```python
from build123d import *

# Parameters (mm, degrees)
SKETCH_1_R          = 3
EXTRUDE_1_DEPTH     = 0.5
SKETCH_2_R          = 1.5
EXTRUDE_2_DEPTH     = 25
CHAMFER_1_SIZE      = 0.2
CUT_EXTRUDE_1_DEPTH = 0.8
FILLET_2_R          = 0.3


with BuildPart() as part:
    # 草图1 → 凸台-拉伸1 (new body, symmetric)
    with BuildSketch(Plane.XY):
        Circle(SKETCH_1_R)
    extrude(amount=EXTRUDE_1_DEPTH, both=True)

    # 草图2 → 凸台-拉伸2 (add)
    with BuildSketch(Plane(origin=(0, 0, -0.5), x_dir=(-1, 0, 0), z_dir=(0, 0, -1))):
        Circle(SKETCH_2_R)
    extrude(amount=EXTRUDE_2_DEPTH)

    # 倒角1
    chamfer_1_edges = [part.edges().sort_by_distance(p)[0] for p in [
        (1.5, 0, -25.5),
    ]]
    chamfer(chamfer_1_edges, length=CHAMFER_1_SIZE)

    # 草图3 → 切除-拉伸1 (cut)
    with BuildSketch(Plane.XY.offset(0.5)):
        Polygon((1.154700538, 0), (0.577350269, 1), (-0.577350269, 1), (-1.154700538, 0), (-0.577350269, -1), (0.577350269, -1), align=None)
    extrude(amount=-CUT_EXTRUDE_1_DEPTH, mode=Mode.SUBTRACT)

    # 圆角2
    fillet_2_edges = [part.edges().sort_by_distance(p)[0] for p in [
        (-3, 0, -0.5),
        (-3, 0, 0.5),
    ]]
    fillet(fillet_2_edges, radius=FILLET_2_R)


solid = part.part
```
The model under review builds one solid part; all positions refer to its coordinate system, in mm. A direction names the side the tool comes from. Coordinates: 2 decimals unless noted, no trailing zeros. Write each loop counter-clockwise with the first axis right and the second up, starting at its lowest first coordinate (ties: lowest second). Pieces come first, ordered by that corner, then holes.
1) We need section B-B on z = -11.5. State the section outline as (x, y) points.
2) Machinability: for faces 4 (the face through (1.2, -1.2, -0.5)), 5 (the face through (0, -1.2, 0.5)), which of the approach directions +Z, -Z, +X, -X, +Y, -Y give a long, thin tool a straight path to every point of the face, cutting with its end or side? Answer none if there is none.
3) We need section A-A on x = 0. State the section outline as (y, z) points, then the cut area to 3 significant figures.
4) Clearance check with flat-ended pins moving along their axes: pin 1 Ø0.6 at (x, y) = (-0.5, 0) entering from +Z; pin 2 Ø1 at (x, z) = (1, -10.5) entering from -Y; pin 3 Ø1 at (y, z) = (-1.5, -17) entering from +X. State where each tip first meets the part, or that it passes through.
5) To check wall thickness, follow probe 1 along Z at (x, y) = (-1.5, 2.25); probe 2 along X at (y, z) = (0.75, -2.25); probe 3 along Z at (x, y) = (1.5, 2.5). State the ranges of each line that lie inside material, in increasing order.
6) The part is to be moulded in two halves that separate along X. For faces 1 (the face through (1.5, 0.07, -12.73)), 2 (the face through (0, 0, -25.5)), 3 (the face through (0, 0, -0.3)), say which applies: pulls with the +X half, pulls with the -X half, needs draft (parallel to the pull), parting line crosses it, or undercut.
Answer list:
1. outline: circle Ø3 at (0, 0)
2. face 4: -Z
2. face 5: +Z, +X, -X, +Y, -Y
3. outline: (-3, -0.2) arc R0.3 ccw to (-2.7, -0.5) - (-1.5, -0.5) - (-1.5, -25.3) - (-1.3, -25.5) - (1.3, -25.5) - (1.5, -25.3) - (1.5, -0.5) - (2.7, -0.5) arc R0.3 ccw to (3, -0.2) - (3, 0.2) arc R0.3 ccw to (2.7, 0.5) - (1, 0.5) - (1, -0.3) - (-1, -0.3) - (-1, 0.5) - (-2.7, 0.5) arc R0.3 ccw to (-3, 0.2) - close
3. area: 79.3 mm2
4. pin 1: stops at z = -0.3
4. pin 2: stops at y = -1.41
4. pin 3: stops at x = 1.12
5. probe 1: z = -0.5 to 0.5
5. probe 2: x = -1.3 to 1.3
5. probe 3: z = -0.41 to 0.41
6. face 1: parting line crosses it
6. face 2: needs draft
6. face 3: undercut
